from build123d import *

# Parameters (mm, degrees)
SKICA1_R                = 1.275
P_IDAT_VYSUNUT_M1_DEPTH = 2.4
ZKOSEN_1_SIZE           = 0.5


with BuildPart() as part:
    # Skica1 → Přidat vysunutím1 (new body)
    with BuildSketch(Plane.XY):
        Polygon((1.517935358, 3.153707699), (-1.972223305, 2.89142443), (-3.490158662, -0.262283268), (-1.517935358, -3.153707699), (1.972223305, -2.89142443), (3.490158662, 0.262283268), align=None)
        Circle(SKICA1_R, mode=Mode.SUBTRACT)
    extrude(amount=P_IDAT_VYSUNUT_M1_DEPTH)

    # Zkosení1
    zkosen_1_edges = [part.edges().sort_by_distance(p)[0] for p in [
        (-1.275, 0, 0),
        (-1.275, 0, 2.4),
    ]]
    chamfer(zkosen_1_edges, length=ZKOSEN_1_SIZE)

    # Skica3 → Odebrat rotací1 (revolve, cut)
    with BuildSketch(Plane(origin=(0, 0, 0), x_dir=(0.9010593425374666, -0.43369581647273064, 0), z_dir=(0.43369581647273064, 0.9010593425374666, 0))):
        Polygon((-5.109549882, 0), (-5.109549882, -1.2), (-3.031088913, 0), align=None)
        Polygon((-5.109549882, -2.4), (-3.031088913, -2.4), (-5.109549882, -1.2), align=None)
    revolve(axis=Axis((0, 0, 2.4), (0, 0, 1)), mode=Mode.SUBTRACT)


solid = part.part
CAD build for the part. Positions are in the model's coordinates, mm. Coordinates: 2 decimals unless noted, no trailing zeros. Write each loop counter-clockwise with the first axis right and the second up, starting at its lowest first coordinate (ties: lowest second). Pieces come first, ordered by that corner, then holes. Notation, with made-up numbers: M 49.5,6.25 L 56.5,6.25 A24 cw 56.5,20.25 Z; hole C 13,31.25 d8. An arc over 180 degrees is marked long. Return JSON: item names as keys, results as strings.
Item 1: Slice it at B-B, the plane y = 0. Write the cut outline in (x, z) (3 decimals), and give its area (3 significant figures).
Findings below:
{"outline": "M -3.364,0.192 L -3.031,0 L -1.775,0 L -1.275,0.5 L -1.275,1.9 L -1.775,2.4 L -3.031,2.4 L -3.364,2.208 Z; M 1.275,0.5 L 1.775,0 L 3.031,0 L 3.364,0.192 L 3.364,2.208 L 3.031,2.4 L 1.775,2.4 L 1.275,1.9 Z", "area": "9.40 mm2"}
Item 2: Two-plate mould, pull along X, no slides. Class faces 1 (the conical face through (1.79, -2.64, 0.09)), 2 (the conical face through (-1.79, 2.64, 0.09)), 3 (the cylindrical face through (0.59, -1.13, 1.19)): +X half, -X half, draft (parallel to the pull), parting line (faces both ways), or undercut.
Findings below:
{"face 1": "+X half", "face 2": "-X half", "face 3": "undercut"}
Item 3: Slice it at A-A, the plane z = 1.15. Write the cut outline in (x, y) (3 decimals), and give its area (3 significant figures).
Findings below:
{"outline": "M -3.49,-0.262 L -1.518,-3.154 L 1.972,-2.891 L 3.49,0.262 L 1.518,3.154 L -1.972,2.891 Z; hole C 0,0 d2.55", "area": "26.7 mm2"}
Item 4: Slice it at C-C, the plane x = 0. Write the cut outline in (y, z) (3 decimals), and give its area (3 significant figures).
Findings below:
{"outline": "M -3.04,0.005 L -3.031,0 L -1.775,0 L -1.275,0.5 L -1.275,1.9 L -1.775,2.4 L -3.031,2.4 L -3.04,2.395 Z; M 1.275,0.5 L 1.775,0 L 3.031,0 L 3.04,0.005 L 3.04,2.395 L 3.031,2.4 L 1.775,2.4 L 1.275,1.9 Z", "area": "7.97 mm2"}
Item 5: Probe line 1 (Y direction, x = 0.75, z = 0.65); line 2 (X direction, y = 1, z = 2.05); line 3 (Y direction, x = 0, z = 1.3) (3 decimals). List the from-to ranges inside material, lowest first. Write a range as from..to.
Findings below:
{"line 1": "y = -2.98..-1.03, 1.03..3.1", "line 2": "x = -2.88..-1.02, 1.02..2.99", "line 3": "y = -3.04..-1.275, 1.275..3.04"}
Item 6: Drop flat-ended pins along their axis: pin 1 Ø1 at (y, z) = (1, 1) entering from -X; pin 2 Ø3.5 at (x, y) = (0, 0) entering from +Z (3 decimals). Give the stop position or say it passes through.
Findings below:
{"pin 1": "stops at x = -3.12", "pin 2": "stops at z = 2.375"}
